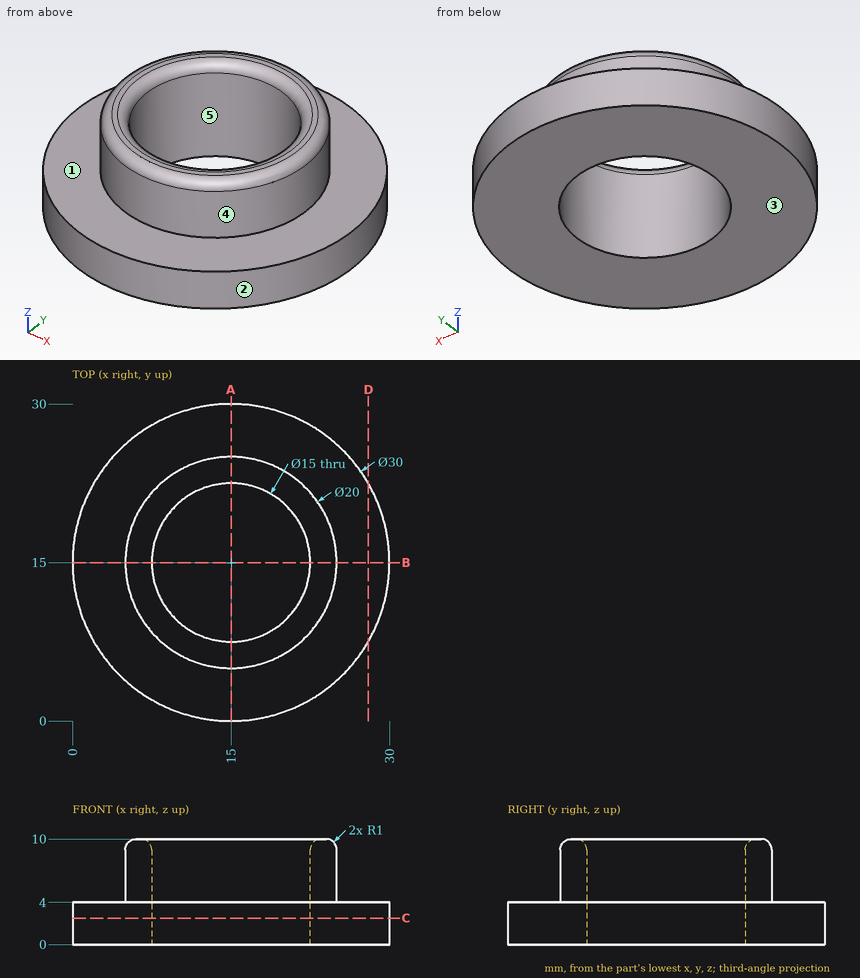
Design review of the part shown in the three views and the two pictorial views. Dimensions are in mm from the part's minimum x, y and z. A direction names the side the tool comes from. Round coordinates to 2 decimals unless told otherwise and drop trailing zeros. Loops run counter-clockwise (first coordinate to the right, second up) from the corner with the lowest first, then second, coordinate; pieces in that order, holes last. Notation, with made-up numbers: (89.25, 17.25) - (102.25, 17.25) arc R17 cw to (102.25, 27.25) - close; hole circle Ø2 at (42, -29.75). An arc over 180 degrees is marked (long way). Use CSV: the item, a comma, the result in double quotes.
(1) Take a section at D-D, the plane x = 28. Give the boundary of the cut face in (y, z).
Working result:
outline,"(7.52, 0) - (22.48, 0) - (22.48, 4) - (7.52, 4) - close"
(2) For line 1 (Y direction, x = 15, z = 2); line 2 (Y direction, x = 16.5, z = 5.5); line 3 (X direction, y = 10.75, z = 4.75), list the stretches that pass through material, from the lowest coordinate up.
Working result:
line 1,"y = 0 to 7.5, 22.5 to 30"
line 2,"y = 5.11 to 7.65, 22.35 to 24.89"
line 3,"x = 5.95 to 8.82, 21.18 to 24.05"
(3) Take a section at A-A, the plane x = 15. Give the boundary of the cut face in (y, z), plus the area to 3 significant figures.
Working result:
outline,"(0, 0) - (7.5, 0) - (7.5, 9) arc R1 ccw to (6.5, 10) - (6, 10) arc R1 ccw to (5, 9) - (5, 4) - (0, 4) - close; (22.5, 0) - (30, 0) - (30, 4) - (25, 4) - (25, 9) arc R1 ccw to (24, 10) - (23.5, 10) arc R1 ccw to (22.5, 9) - close"
area,"89.1 mm^2"
(4) The part is to be moulded in two halves that separate along X. For the marked faces 3, 4 and 5, say which applies: pulls with the +X half, pulls with the -X half, needs draft (parallel to the pull), parting line crosses it, or undercut.
Working result:
face 3,"needs draft"
face 4,"parting line crosses it"
face 5,"undercut"
(5) Machinability: for the marked faces 1 and 2, which of the approach directions +Z, -Z, +X, -X, +Y, -Y give a long, thin tool a straight path to every point of the face, cutting with its end or side? Answer none if there is none.
Working result:
face 1,"+Z"
face 2,"+Z, -Z"
(6) Take a section at C-C, the plane z = 2.5. Give the boundary of the cut face in (x, y).
Working result:
outline,"circle Ø30 at (15, 15); hole circle Ø15 at (15, 15)"
(7) Clearance check with flat-ended pins moving along their axes: P1, Ø1, axis at y = 7.5, z = 3.5, coming from the +X side; P2, Ø5, axis at y = 21, z = 7, coming from the +X side; P3, Ø1.5, axis at y = 13.5, z = 3.5, coming from the +X side. State where each tip first meets the part, or that it passes through.
Working result:
P1,"stops at x = 28.27"
P2,"stops at x = 24.37"
P3,"stops at x = 29.98"
